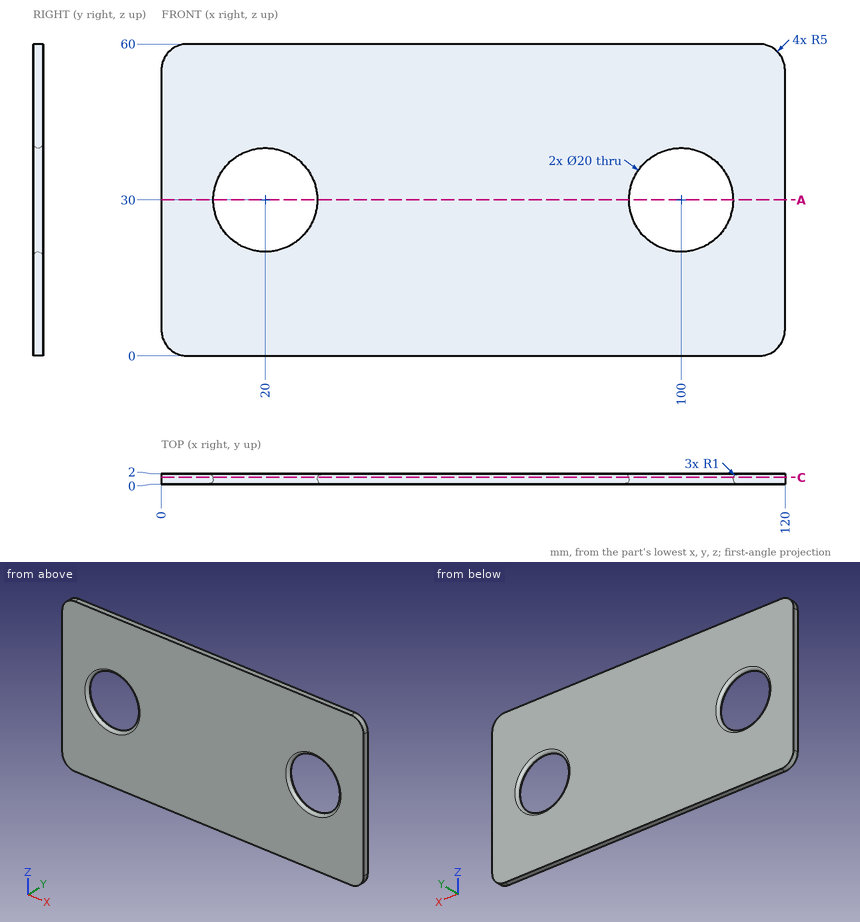
Could you check a few things on this drawing? It's one solid part, dimensions in mm from its lowest x, y, z. Coordinates: 2 decimals unless noted, no trailing zeros. Order: outer loops, then holes, each group sorted by start corner. A loop starts at its lowest first (then second) coordinate and runs counter-clockwise, first axis right, second up.
1. If we section it at A-A (z = 30): Give the number of separate pieces and of enclosed holes in the cut face, then the cut area to 3 significant figures.
2. If we section it at C-C (y = 1.3): Please give me the cut outline in (x, z), then the cut area to 3 significant figures.
3. I need wall thicknesses on line 1 (X direction, y = 1.05, z = 30); line 2 (X direction, y = 0.35, z = 31); line 3 (Z direction, x = 24, y = 1.35). Which ranges of each line are inside material? Lowest first, please.
4. I'm going to push a flat-ended pin straight in: pin 1 (18 mm diameter, centred on x = 100, z = 30, fed in from +Y). Where does the tip first touch, or does it pass through?
Entries:
1. separate pieces: 3
1. enclosed holes: 0
1. area: 158 mm2
2. outline: (0, 5) arc R5 ccw to (5, 0) - (115, 0) arc R5 ccw to (120, 5) - (120, 55) arc R5 ccw to (115, 60) - (5, 60) arc R5 ccw to (0, 55) - close; hole circle Ø20.09 at (20, 30); hole circle Ø20.09 at (100, 30)
2. area: 6,540 mm2
3. line 1: x = 0 to 10, 30 to 90, 110 to 120
3. line 2: x = 0 to 9.81, 30.19 to 89.81, 110.19 to 120
3. line 3: z = 0 to 20.77, 39.23 to 60
4. pin 1: passes through
